The figure shows three views and two pictorial views of one solid part (mm, origin at its lowest corner). Answer the questions. Round coordinates to 2 decimals unless told otherwise and drop trailing zeros. Order: outer loops, then holes, each group sorted by start corner. A loop starts at its lowest first (then second) coordinate and runs counter-clockwise, first axis right, second up. Notation, with made-up numbers: (-27.5, 70.25) - (27.5, 70.25) arc R22 ccw to (27.5, 77.25) - close; hole circle Ø6 at (16, 20). An arc over 180 degrees is marked (long way). Answer as a JSON object with one key per item and string values. Group by question number.
Q1. Consider line 1 (X direction, y = 3.5, z = 3.7) (1 decimal); line 2 (X direction, y = 4.1, z = 1.9) (1 decimal); line 3 (Y direction, x = 1.8, z = 5.7) (1 decimal). Determine where each line is inside the solid, lowest interval first.
Q2. A cutting plane is placed at A-A on z = 4. Determine the outline of the cut face in (x, y).
Q3. The mould has two halves that part along Y. Classify the marked faces 1, 2 and 3: pulls with the +Y half, pulls with the -Y half, needs draft (parallel to the pull), parting line crosses it, or undercut.
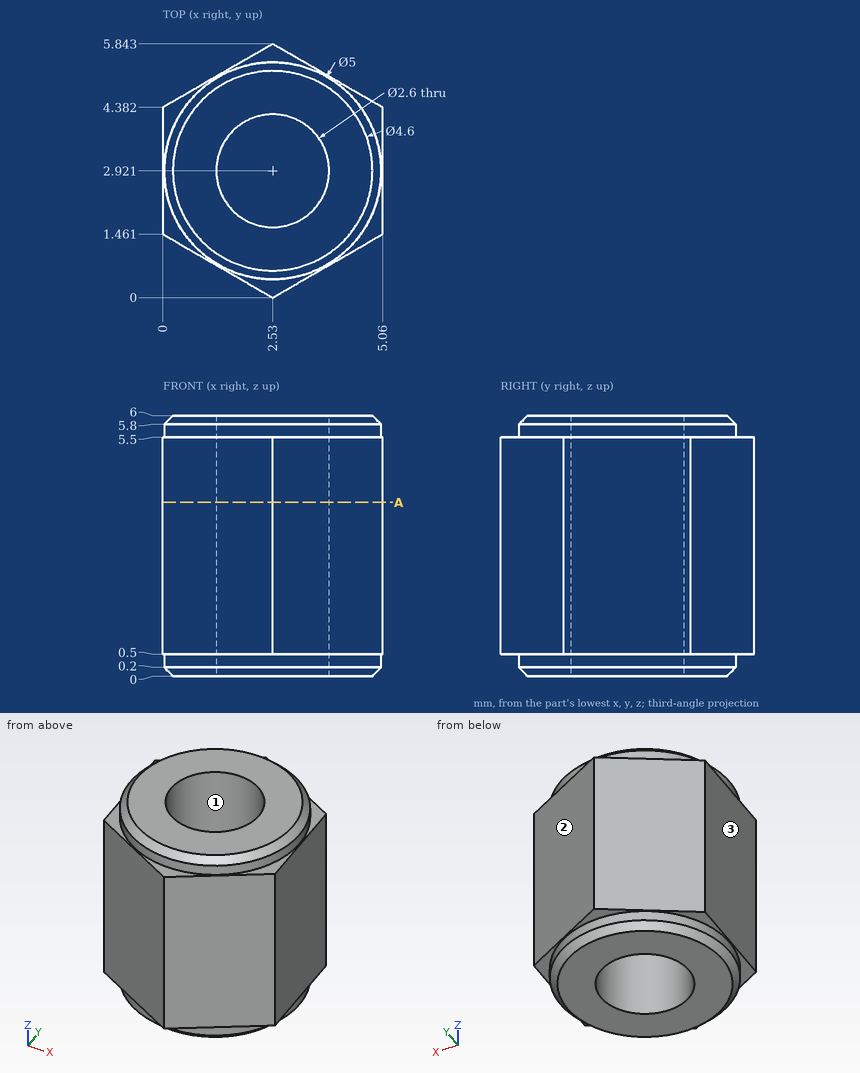
Result set:
{
 "1": {"line 1": "x = 0 to 1.4, 3.7 to 5.1", "line 2": "x = 0 to 2, 3.1 to 5.1", "line 3": "y = 0.5 to 1.8, 4 to 5.3"},
 "2": {"outline": "(0, 1.46) - (2.53, 0) - (5.06, 1.46) - (5.06, 4.38) - (2.53, 5.84) - (0, 4.38) - close; hole circle Ø2.6 at (2.53, 2.92)"},
 "3": {"face 1": "undercut", "face 2": "pulls with the +Y half", "face 3": "needs draft"}
}
